Build history of the part. All positions in model axes, mm. A direction names the side the tool comes from. Coordinates: 2 decimals unless noted, no trailing zeros. Loops run counter-clockwise (first coordinate to the right, second up) from the corner with the lowest first, then second, coordinate; pieces in that order, holes last.
Item 1: Drill centre lines: line 1 along Z through (x, y) = (0, 10.25); line 2 along Y through (x, z) = (31.5, 21); line 3 along Y through (x, z) = (9.5, 2.5). Where is each one in solid material? Low to high.
Item 2: Cut at C-C (y = 9). List the corners of the cut face in (x, z).
Item 3: Cut at D-D (x = -19). List the corners of the cut face in (y, z), and give its area (3 significant figures).
Item 4: 3-axis set-ups, long thin cutter, end or side, ignore diameter. For faces 1 (the face through (-6, 25, -30)), 2 (the face through (0, 17, 0)), 3 (the face through (17, 0, -1)): which of +Z, -Z, +X, -X, +Y, -Y reach the whole face in a straight line?
Item 5: Cut at B-B (z = 0). List the corners of the cut face in (x, y), and give its area (3 significant figures).
Item 6: Flat gauge pins, fed straight in: pin 1 (1 mm diameter, centred on x = 22, y = 16.5, fed in from -Z); pin 2 (8.5 mm diameter, centred on x = 2, z = 0, fed in from -Y); pin 3 (12 mm diameter, centred on y = 19.5, z = -19.5, fed in from -X). Where does each tip first touch, or does it go through?
Item 7: Cut at A-A (x = 0). List the corners of the cut face in (y, z), and give its area (3 significant figures).
Item 8: Mould opens along Z. For faces 4 (the face through (0, 30, 0)), 5 (the face through (-29.97, 27.46, -1.32)), 6 (the face through (12.932, 8.381, -5.362)) say: released by +Z, released by -Z, zero draft, split by the parting line, or undercut.
from build123d import *

# Parameters (mm, degrees)
SKETCH2_R          = 14
CUT_EXTRUDE1_DEPTH = 17


with BuildPart() as part:
    # Sketch1 → Revolve1 (revolve)
    with BuildSketch(Plane.XY):
        Polygon((0, 0), (0, 30), (30, 30), (30, 25), (40, 25), (40, 0), align=None)
    revolve(axis=Axis((0, 0, 0), (0, 1, 0)))

    # Sketch2 → Cut-Extrude1 (cut)
    with BuildSketch(Plane.XZ):
        Circle(SKETCH2_R)
    extrude(amount=-CUT_EXTRUDE1_DEPTH, mode=Mode.SUBTRACT)


solid = part.part
Filled sheet:
1. line 1: z = -40 to -14, 14 to 40
1. line 2: y = 0 to 25
1. line 3: y = 17 to 30
2. outline: circle Ø80 at (0, 0); hole circle Ø28 at (0, 0)
3. outline: (0, -35.2) - (25, -35.2) - (25, -23.22) - (30, -23.22) - (30, 23.22) - (25, 23.22) - (25, 35.2) - (0, 35.2) - close
3. area: 1,990 mm2
4. face 1: +Y
4. face 2: -Y
4. face 3: +Z, -Z, +X, -X, -Y
5. outline: (-40, 0) - (-14, 0) - (-14, 17) - (14, 17) - (14, 0) - (40, 0) - (40, 25) - (30, 25) - (30, 30) - (-30, 30) - (-30, 25) - (-40, 25) - close
5. area: 1,820 mm2
6. pin 1: stops at z = -33.73
6. pin 2: stops at y = 17
6. pin 3: stops at x = -37.65
7. outline: (0, -40) - (25, -40) - (25, -30) - (30, -30) - (30, 30) - (25, 30) - (25, 40) - (0, 40) - (0, 14) - (17, 14) - (17, -14) - (0, -14) - close
7. area: 1,820 mm2
8. face 4: zero draft
8. face 5: split by the parting line
8. face 6: undercut
